Autodesk Inventor part; units mm, degrees
ref_plane "YZ Plane" through (0, 0, 0) normal (1, 0, 0) x (0, 1, 0)
ref_plane "XZ Plane" through (0, 0, 0) normal (0, 1, 0) x (-1, 0, 0)
ref_plane "XY Plane" through (0, 0, 0) normal (0, 0, 1) x (1, 0, 0)
sketch "Sketch1" plane through (0, 0, 0) normal (0, 1, 0) x (-1, 0, 0)
  line L0 (-10, -20) -> (10, -20)
  line L1 (10, -20) -> (10, 20)
  line L2 (10, 20) -> (-10, 20)
  line L3 (-10, 20) -> (-10, -20)
  line L4 (-10, -20) -> (10, 20) construction
  line L5 (10, -20) -> (-10, 20) construction
  point P0 (0, 0)
  dimension "d0" = 20
  dimension "d1" = 40
extrude "Extrusion1" add sketch "Sketch1" along normal blind 85
sketch "Sketch2" plane through (0, 0, 0) normal (0, -1, 0) x (1, 0, 0)
  line L0 (10, -20) -> (-10, -20)
  line L1 (10, 20) -> (10, -20)
  line L2 (-10, 20) -> (10, 20)
  line L3 (-10, -20) -> (-10, 20)
  line L4 (10, 20) -> (10, -20)
  line L5 (10, 18.3) -> (-5.8, 18.3)
  line L6 (-5.8, 18.3) -> (-5.8, 16.1)
  line L7 (-5.8, 16.1) -> (10, 16.1)
  line L8 (10, 16.1) -> (10, 18.3)
  point P0 (0, 0)
  dimension "d4" = 1.7
  dimension "d5" = 4.2
  dimension "d6" = 2.2
extrude "Extrusion2" cut sketch "Sketch2" against normal through all contours L7 L6 L5 L1
mirror "Mirror1" about plane through (0, 0, 0) normal (0, 0, 1) of "Extrusion2"
sketch "Sketch3" plane through (0, 0, 0) normal (0, -1, 0) x (1, 0, 0)
  line L0 (-5.8, -16.1) -> (10, -16.1)
  line L1 (10, 16.1) -> (10, -16.1)
  line L2 (10, 16.1) -> (-5.8, 16.1)
  line L3 (-5.8, 16.1) -> (-5.8, 18.3)
  line L4 (-5.8, 18.3) -> (10, 18.3)
  line L5 (10, 20) -> (10, 18.3)
  line L6 (-10, 20) -> (10, 20)
  line L7 (-10, -20) -> (-10, 20)
  line L8 (10, -20) -> (-10, -20)
  line L9 (10, -18.3) -> (10, -20)
  line L10 (10, -18.3) -> (-5.8, -18.3)
  line L11 (-5.8, -18.3) -> (-5.8, -16.1)
  line L12 (10, 14.8) -> (-5.8, 14.8)
  line L13 (-5.8, 14.8) -> (-5.8, 12.28)
  line L14 (-5.8, 12.28) -> (10, 12.28)
  line L15 (10, 12.28) -> (10, 14.8)
  point P0 (0, 0)
  dimension "d9" = 1.3
  dimension "d10" = 2.52
extrude "Extrusion3" cut sketch "Sketch3" against normal through all contours L14 L13 L12 L1
pattern_linear "Rectangular Pattern1" count 8 spacing 3.82 along (0, 0, -1) of "Extrusion3"
sketch "Sketch4" plane through (-10, 0, -20) normal (-1, 0, 0) x (0, 0, 1)
  line L0 (0, 0) -> (40, 0)
  line L1 (40, 0) -> (40, 85)
  line L2 (0, 85) -> (40, 85)
  line L3 (0, 0) -> (0, 85)
  point P0 (20, 0)
extrude "Extrusion4" cut sketch "Sketch4" against normal blind 2
sketch "Sketch5" plane through (10, 0, 20) normal (1, 0, 0) x (0, 0, -1)
  line L0 (-7.9901, -7.3422) -> (53.3048, -7.3422)
  line L1 (53.3048, -7.3422) -> (53.3048, 101.8937)
  line L2 (53.3048, 101.8937) -> (-7.9901, 101.8937)
  line L3 (-7.9901, 101.8937) -> (-7.9901, -7.3422)
  point P0 (20, 0)
extrude "Extrusion5" cut sketch "Sketch5" against normal blind 8
sketch "Sketch7" plane through (-8, 0, -20) normal (-1, 0, 0) x (0, 0, 1)
  circle A0 centre (37, 26) radius 4.7625
  line L0 (40, 85) -> (40, 0)
  line L1 (40, 0) -> (0, 0)
  line L2 (37, 21.2375) -> (47, 21.2375)
  line L3 (47, 21.2375) -> (47, 30.7625)
  line L4 (47, 30.7625) -> (37, 30.7625)
  line L5 (37, 30.7625) -> (37, 21.2375)
  point P0 (20, 0)
  dimension "d24" = 9.525
  dimension "d25" = 3
  dimension "d26" = 26
  dimension "d29" = 10
extrude "Extrusion7" cut sketch "Sketch7" against normal blind 1
properties part number "Ultra96_Heatsink"
Geometry: final body of the model. Coordinates: model frame, mm. A direction names the side the tool comes from. Round coordinates to 2 decimals unless told otherwise and drop trailing zeros. Write item = value, one per line.
Item 1: Pull-direction query (Y, two-part tool) for faces 3 (the face through (-2, 42, 4.64)), 4 (the face through (-7, 26, 17)); classes: pulls with the +Y half, pulls with the -Y half, needs draft (parallel to the pull), parting line crosses it, or undercut.
Findings:
face_3 = needs draft
face_4 = undercut
Item 2: Section query A-A on x = 0.25. State how many separate pieces and enclosed holes the cut face has, then the cut area to 3 significant figures.
Findings:
separate_pieces = 11
enclosed_holes = 0
area = 1,310 mm^2
Item 3: Material intervals for line 1 along X through (y, z) = (28.5, -1.5), sorted ascending. Write a range as [from, to].
Findings:
line_1 = [-8, -5.8]
Item 4: Pin query (flat end, axial travel): P1, Ø1.5, axis at x = -2, z = -9.5, coming from the +Y side; P2, Ø0.8, axis at y = 52, z = -9.5, coming from the +X side. Return the tip coordinate at first contact, or that it passes through.
Findings:
P1 = through
P2 = -5.8
Item 5: Access query for faces 1 (the face through (-2, 42, 16.1)), 2 (the face through (-3, 42, 20)). Directions: +Z, -Z, +X, -X, +Y, -Y. A direction counts if a zero-diameter tool reaches every point of the face in a straight line with its end or side. Return the directions, or none.
Findings:
face_1 = +X, +Y, -Y
face_2 = +Z, +X, -X, +Y, -Y
